For this review, use the dimensioned drawing (mm, ordinates from the lowest corner) and the shaded views. A direction names the side the tool comes from. Coordinates: 2 decimals unless noted, no trailing zeros. Loops run counter-clockwise (first coordinate to the right, second up) from the corner with the lowest first, then second, coordinate; pieces in that order, holes last. Notation, with made-up numbers: M 4.5,16.25 L 43.5,16.25 A22 cw 43.5,35.25 Z; hole C -2,72 d3. An arc over 180 degrees is marked long. One line per item, written item: value.
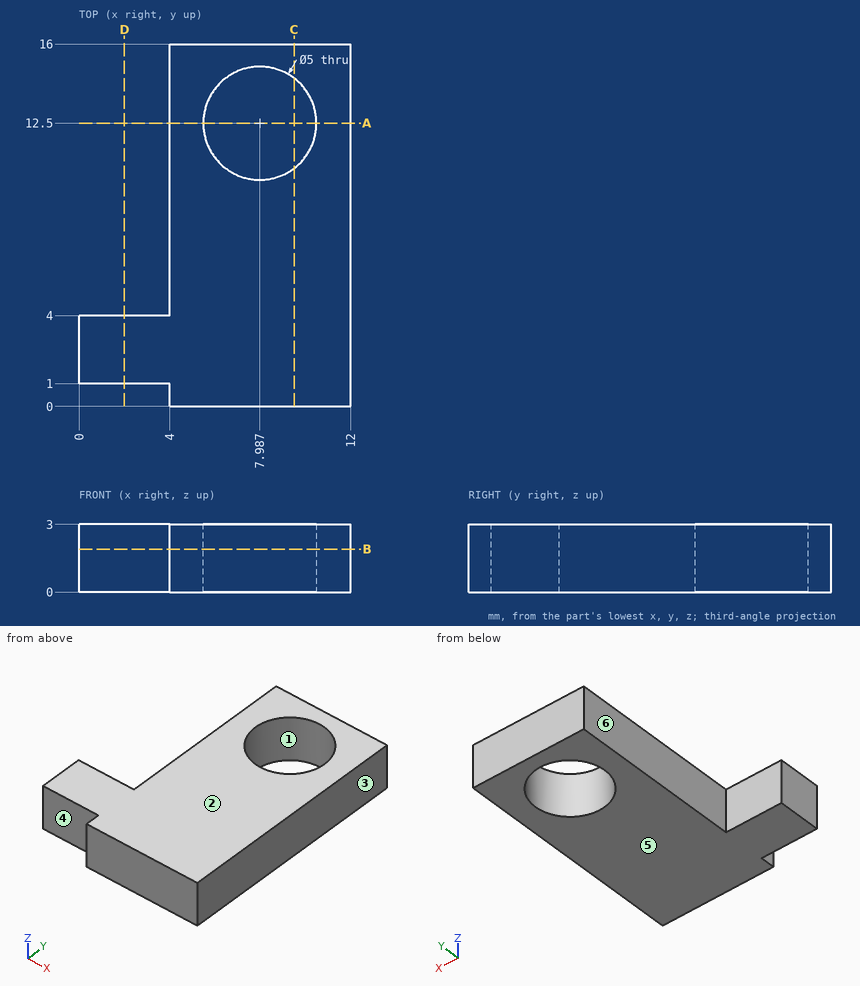
(1) We need section D-D on x = 2. State the section outline as (y, z) points.
Reply:
outline: M 1,0 L 4,0 L 4,3 L 1,3 Z
(2) We need section B-B on z = 1.9. State the section outline as (x, y) points, then the cut area to 3 significant figures.
Reply:
outline: M 0,1 L 4,1 L 4,0 L 12,0 L 12,16 L 4,16 L 4,4 L 0,4 Z; hole C 7.99,12.5 d5
area: 120 mm2
(3) Insertion check: pin 1 (0.8 mm diameter, centred on y = 0.5, z = 2, fed in from -X); pin 2 (0.9 mm diameter, centred on x = 1, z = 1, fed in from +Y); pin 3 (1.5 mm diameter, centred on x = 2.5, z = 0.5, fed in from -Y). Each pin has a flat end and moves straight along its axis. Give the tip position at first contact, or say it passes through.
Reply:
pin 1: stops at x = 4
pin 2: stops at y = 4
pin 3: stops at y = 1
(4) Mouldability with a two-part tool opening along X and no side actions: class the marked faces 1, 2 and 3 as released by +X, released by -X, zero draft, split by the parting line, or undercut.
Reply:
face 1: undercut
face 2: zero draft
face 3: released by +X
(5) To check wall thickness, follow line 1 along X through (y, z) = (7.25, 1.5); line 2 along Y through (x, z) = (2.25, 1.75); line 3 along Y through (x, z) = (7.5, 1.65). State the ranges of each line that lie inside material, in increasing order. Write a range as [from, to].
Reply:
line 1: x = [4, 12]
line 2: y = [1, 4]
line 3: y = [0, 10.05], [14.95, 16]
(6) Tool access review of the marked faces 4, 5 and 6: name each direction out of +Z, -Z, +X, -X, +Y, -Y from which nothing blocks a thin tool from reaching the whole face with its end or side.
Reply:
face 4: +Z, -Z, -X, -Y
face 5: -Z, +X, -X, +Y, -Y
face 6: +Z, -Z, -X, +Y
(7) We need section C-C on x = 9.5. State the section outline as (y, z) points.
Reply:
outline: M 0,0 L 10.51,0 L 10.51,3 L 0,3 Z; M 14.49,0 L 16,0 L 16,3 L 14.49,3 Z
(8) We need section A-A on y = 12.5. State the section outline as (x, z) points.
Reply:
outline: M 4,0 L 5.49,0 L 5.49,3 L 4,3 Z; M 10.49,0 L 12,0 L 12,3 L 10.49,3 Z
